Part print with two shaded views. Sizes in mm from the minimum x, y, z corner. A direction names the side the tool comes from. Give positions to 0.01 mm unless a question says otherwise; leave off trailing zeros. Order: outer loops, then holes, each group sorted by start corner. A loop starts at its lowest first (then second) coordinate and runs counter-clockwise, first axis right, second up. Notation, with made-up numbers: (77.25, 31.25) - (95.25, 31.25) arc R24 ccw to (95.25, 42.25) - close; hole circle Ø6 at (1, -39.5). An arc over 180 degrees is marked (long way). Return JSON: item names as keys, results as strings. Group by question number.
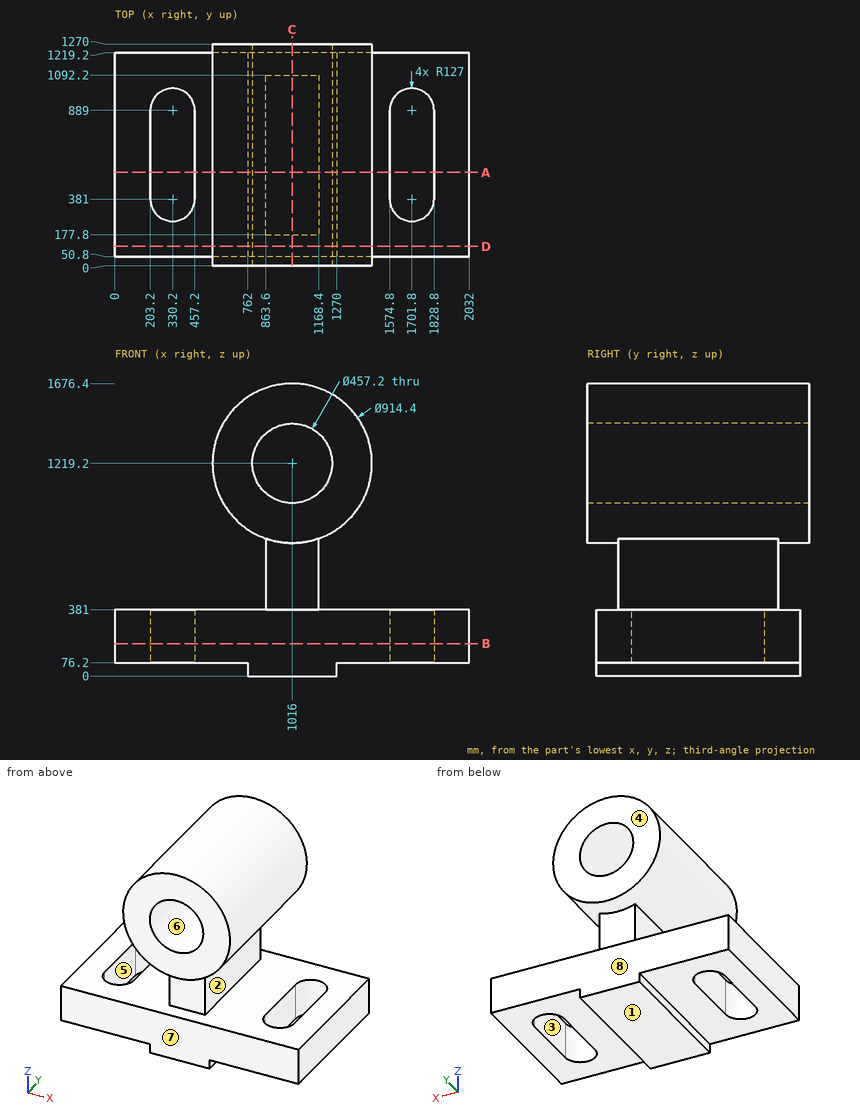
(1) 3-axis set-ups, long thin cutter, end or side, ignore diameter. For the marked faces 4, 5, 6, 7 and 8: which of +Z, -Z, +X, -X, +Y, -Y reach the whole face in a straight line?
(2) Drop flat-ended pins along their axis: pin 1 Ø6 at (y, z) = (937, 1296) entering from -X; pin 2 Ø6 at (x, y) = (272.5, 1032) entering from -Z; pin 3 Ø8 at (y, z) = (189, 469.5) entering from +X. Give the stop position or say it passes through.
(3) Slice it at D-D (y = 110.5). Give the cut face in (x, z), and give its area (3 significant figures).
(4) Slice it at B-B (z = 185.5). Give the cut face in (x, y).
(5) Slice it at C-C (x = 1016). Give the cut face in (y, z), and give its area (3 significant figures).
(6) Drill centre lines: L1, parallel to X at y = 552.5, z = 96; L2, parallel to X at y = 893.5, z = 1219.2; L3, parallel to Y at x = 1422, z = 187.5. Where is each one in solid material? Low to high.
(7) Slice it at A-A (y = 534). Give the cut face in (x, z), and give its area (3 significant figures).
(8) Pull direction Z, two halves, no side cores. Call the marked faces 1, 2 and 3: released by +Z, released by -Z, zero draft, split by the parting line, or undercut.
Result set:
{
 "1": {"face 4": "+Z, -Z, +X, -X, +Y", "face 5": "+Z, -Z", "face 6": "+Y, -Y", "face 7": "-Z, +X, -X, -Y", "face 8": "-Z, +X, -X, +Y"},
 "2": {"pin 1": "stops at x = 564.8", "pin 2": "stops at z = 76.2", "pin 3": "stops at x = 1168.4"},
 "3": {"outline": "(0, 76.2) - (762, 76.2) - (762, 0) - (1270, 0) - (1270, 76.2) - (2032, 76.2) - (2032, 381) - (0, 381) - close; circle Ø914.4 at (1016, 1219.2); hole circle Ø457.2 at (1016, 1219.2)", "area": "1,150,000 mm²"},
 "4": {"outline": "(0, 50.8) - (2032, 50.8) - (2032, 1219.2) - (0, 1219.2) - close; hole (203.2, 381) arc R127 ccw to (457.2, 381) - (457.2, 889) arc R127 ccw to (203.2, 889) - close; hole (1574.8, 381) arc R127 ccw to (1828.8, 381) - (1828.8, 889) arc R127 ccw to (1574.8, 889) - close"},
 "5": {"outline": "(0, 762) - (177.8, 762) - (177.8, 381) - (50.8, 381) - (50.8, 0) - (1219.2, 0) - (1219.2, 381) - (1092.2, 381) - (1092.2, 762) - (1270, 762) - (1270, 990.6) - (0, 990.6) - close; (0, 1447.8) - (1270, 1447.8) - (1270, 1676.4) - (0, 1676.4) - close", "area": "1,370,000 mm²"},
 "6": {"L1": "x = 0 to 203.2, 457.2 to 1574.8, 1828.8 to 2032", "L2": "x = 558.8 to 787.4, 1244.6 to 1473.2", "L3": "y = 50.8 to 1219.2"},
 "7": {"outline": "(0, 76.2) - (203.2, 76.2) - (203.2, 381) - (0, 381) - close; (457.2, 76.2) - (762, 76.2) - (762, 0) - (1270, 0) - (1270, 76.2) - (1574.8, 76.2) - (1574.8, 381) - (1168.4, 381) - (1168.4, 788.15) arc R457.2 ccw (long way) to (863.6, 788.15) - (863.6, 381) - (457.2, 381) - close; (1828.8, 76.2) - (2032, 76.2) - (2032, 381) - (1828.8, 381) - close; hole circle Ø457.2 at (1016, 1219.2)", "area": "1,110,000 mm²"},
 "8": {"face 1": "released by -Z", "face 2": "undercut", "face 3": "zero draft"}
}
